For this review, take the finished solid that the model builds, in its own axes (mm). Coordinates: 2 decimals unless noted, no trailing zeros. Loops run counter-clockwise (first coordinate to the right, second up) from the corner with the lowest first, then second, coordinate; pieces in that order, holes last. Notation, with made-up numbers: (67.5, -31) - (81.5, -31) arc R24 ccw to (81.5, -14) - close; hole circle Ø3 at (35.25, -18.5). An arc over 180 degrees is marked (long way). Answer as a JSON object with one key per item and string values. Group by question number.
Item 1: To check wall thickness, follow line 1 (X direction, y = 1.15, z = -39); line 2 (Z direction, x = -18.5, y = 1.3); line 3 (X direction, y = 2.6, z = 25). State the ranges of each line that lie inside material, in increasing order.
Item 2: Clearance check with a flat-ended pin moving along its axis: pin 1 (1.5 mm diameter, centred on x = 70.5, y = 1, fed in from -Z). State where the tip first meets the part, or that it passes through.
Item 3: We need section B-B (y = 1.1). State how many separate pieces and enclosed holes the cut face has, then the cut area to 3 significant figures.
Item 4: We need section A-A (z = 12). Give the boundary of the cut face in (x, y).
from build123d import *

# Parameters (mm, degrees)
SKETCH1_R                = 100
SKETCH1_R_2              = 5
BOSS_EXTRUDE1_DEPTH      = 3
SKETCH2_W                = 5.2
SKETCH2_H                = 2.7
CUT_EXTRUDE1_DEPTH       = 4
CUT_EXTRUDE2_DEPTH       = 4
SKETCH4_W                = 5
SKETCH4_H                = 60
CUT_EXTRUDE3_DEPTH       = 4
FILLET3_R                = 10
FILLET2_R                = 1
SKETCH5_R                = 1.075
CUT_EXTRUDE4_DEPTH       = 4
SKETCH6_R                = 9
SKETCH6_R_2              = 1.1
CUT_EXTRUDE5_DEPTH       = 4
IR_HOLDER_HOLES_REACH    = 5
IR_HOLDER_HOLES_SKETCH_R = 1.5
PLATFORM_HOLES_REACH     = 5
PLATFORM_HOLES_SKETCH_R  = 1.5


with BuildPart() as part:
    # Sketch1 → Boss-Extrude1 (new body)
    with BuildSketch(Plane(origin=(0, 0, 0), x_dir=(1, 0, 0), z_dir=(0, 1, 0))):
        Circle(SKETCH1_R)
        Circle(SKETCH1_R_2, mode=Mode.SUBTRACT)
    extrude(amount=BOSS_EXTRUDE1_DEPTH)

    # Sketch2 → Cut-Extrude1 (cut, through all)
    with BuildSketch(Plane(origin=(0, 3, 0), x_dir=(1, 0, 0), z_dir=(0, 1, 0))):
        with Locations((-54.5, 37.95)):
            Rectangle(SKETCH2_W, SKETCH2_H)
        with Locations((-54.5, 28.45)):
            Rectangle(SKETCH2_W, SKETCH2_H)
        with Locations((-54.5, 4.75)):
            Rectangle(SKETCH2_W, SKETCH2_H)
        with Locations((-54.5, -4.75)):
            Rectangle(SKETCH2_W, SKETCH2_H)
        with Locations((-77.5, -4.75)):
            Rectangle(SKETCH2_W, SKETCH2_H)
        with Locations((-77.5, 4.75)):
            Rectangle(SKETCH2_W, SKETCH2_H)
        with Locations((54.5, 28.45)):
            Rectangle(SKETCH2_W, SKETCH2_H)
        with Locations((54.5, 37.95)):
            Rectangle(SKETCH2_W, SKETCH2_H)
        with Locations((77.5, 4.75)):
            Rectangle(SKETCH2_W, SKETCH2_H)
        with Locations((77.5, -4.75)):
            Rectangle(SKETCH2_W, SKETCH2_H)
        with Locations((54.5, -4.75)):
            Rectangle(SKETCH2_W, SKETCH2_H)
        with Locations((54.5, 4.75)):
            Rectangle(SKETCH2_W, SKETCH2_H)
    extrude(amount=-CUT_EXTRUDE1_DEPTH, mode=Mode.SUBTRACT)

    # Sketch3 → Cut-Extrude2 (cut, through all)
    with BuildSketch(Plane(origin=(0, 3, 0), x_dir=(1, 0, 0), z_dir=(0, 1, 0))):
        with BuildLine():
            ThreePointArc((67.534713296, 73.75), (0, 100), (-67.534713296, 73.75))
            Line((-67.534713296, 73.75), (67.534713296, 73.75))
        make_face()
        with BuildLine():
            Line((-85.1, -52.516568814), (-85.1, 52.516568814))
            ThreePointArc((-85.1, 52.516568814), (-100, 0), (-85.1, -52.516568814))
        make_face()
        with BuildLine():
            Line((67.534713296, -73.75), (-67.534713296, -73.75))
            ThreePointArc((-67.534713296, -73.75), (0, -100), (67.534713296, -73.75))
        make_face()
        with BuildLine():
            ThreePointArc((100, 0), (96.202910559, 27.294688128), (85.1, 52.516568814))
            Line((85.1, 52.516568814), (85.1, -52.516568814))
            ThreePointArc((85.1, -52.516568814), (96.202910559, -27.294688128), (100, 0))
        make_face()
    extrude(amount=-CUT_EXTRUDE2_DEPTH, mode=Mode.SUBTRACT)

    # Sketch4 → Cut-Extrude3 (cut, through all)
    with BuildSketch(Plane(origin=(0, 3, 0), x_dir=(1, 0, 0), z_dir=(0, 1, 0))):
        with Locations((-70.7, 0)):
            Rectangle(SKETCH4_W, SKETCH4_H)
        with Locations((70.7, 0)):
            Rectangle(SKETCH4_W, SKETCH4_H)
    extrude(amount=-CUT_EXTRUDE3_DEPTH, mode=Mode.SUBTRACT)

    # Fillet3
    fillet3_edges = [part.edges().sort_by_distance(p)[0] for p in [
        (-67.534713296, 1.5, -73.75),
        (67.534713296, 1.5, -73.75),
        (-85.1, 1.5, -52.516568814),
        (-85.1, 1.5, 52.516568814),
        (-67.534713296, 1.5, 73.75),
        (67.534713296, 1.5, 73.75),
        (85.1, 1.5, -52.516568814),
        (85.1, 1.5, 52.516568814),
    ]]
    fillet(fillet3_edges, radius=FILLET3_R)

    # Fillet2
    fillet2_edges = [part.edges().sort_by_distance(p)[0] for p in [
        (-73.2, 1.5, 30),
        (-73.2, 1.5, -30),
        (-68.2, 1.5, -30),
        (-68.2, 1.5, 30),
        (73.2, 1.5, -30),
        (73.2, 1.5, 30),
        (68.2, 1.5, 30),
        (68.2, 1.5, -30),
    ]]
    fillet(fillet2_edges, radius=FILLET2_R)

    # Sketch5 → Cut-Extrude4 (cut, through all)
    with BuildSketch(Plane(origin=(0, 3, 0), x_dir=(1, 0, 0), z_dir=(0, 1, 0))):
        with Locations((-54.5, 33.2)):
            Circle(SKETCH5_R)
        with Locations((-54.5, 0)):
            Circle(SKETCH5_R)
        with Locations((-77.5, 0)):
            Circle(SKETCH5_R)
        with Locations((77.5, 0)):
            Circle(SKETCH5_R)
        with Locations((54.5, 0)):
            Circle(SKETCH5_R)
        with Locations((54.5, 33.2)):
            Circle(SKETCH5_R)
    extrude(amount=-CUT_EXTRUDE4_DEPTH, mode=Mode.SUBTRACT)

    # Sketch6 → Cut-Extrude5 (cut, through all)
    with BuildSketch(Plane(origin=(0, 3, 0), x_dir=(1, 0, 0), z_dir=(0, 1, 0))):
        with Locations((0, 57.75)):
            Circle(SKETCH6_R)
        with Locations((0, 69.75)):
            Circle(SKETCH6_R_2)
        with Locations((12, 57.75)):
            Circle(SKETCH6_R_2)
        with Locations((0, 45.75)):
            Circle(SKETCH6_R_2)
        with Locations((-12, 57.75)):
            Circle(SKETCH6_R_2)
        with Locations((-12, -57.75)):
            Circle(SKETCH6_R_2)
        with Locations((0, -45.75)):
            Circle(SKETCH6_R_2)
        with Locations((12, -57.75)):
            Circle(SKETCH6_R_2)
        with Locations((0, -69.75)):
            Circle(SKETCH6_R_2)
        with Locations((0, -57.75)):
            Circle(SKETCH6_R)
    extrude(amount=-CUT_EXTRUDE5_DEPTH, mode=Mode.SUBTRACT)

    # IR Holder Holes Sketch → IR Holder Holes (cut, up to next)
    with BuildSketch(Plane(origin=(0, 3, 0), x_dir=(1, 0, 0), z_dir=(0, 1, 0)), mode=Mode.PRIVATE) as ir_holder_holes_sk1:
        with Locations((18.5, -65.75)):
            Circle(IR_HOLDER_HOLES_SKETCH_R)
    ir_holder_holes_tool1 = extrude(ir_holder_holes_sk1.sketch, amount=-IR_HOLDER_HOLES_REACH, mode=Mode.PRIVATE) & part.part
    add(ir_holder_holes_tool1.solids().sort_by_distance((18.5, 3, 65.75))[0], mode=Mode.SUBTRACT)
    # IR Holder Holes Sketch → IR Holder Holes (cut, up to next)
    with BuildSketch(Plane(origin=(0, 3, 0), x_dir=(1, 0, 0), z_dir=(0, 1, 0)), mode=Mode.PRIVATE) as ir_holder_holes_sk2:
        with Locations((18.5, -49.75)):
            Circle(IR_HOLDER_HOLES_SKETCH_R)
    ir_holder_holes_tool2 = extrude(ir_holder_holes_sk2.sketch, amount=-IR_HOLDER_HOLES_REACH, mode=Mode.PRIVATE) & part.part
    add(ir_holder_holes_tool2.solids().sort_by_distance((18.5, 3, 49.75))[0], mode=Mode.SUBTRACT)
    # IR Holder Holes Sketch → IR Holder Holes (cut, up to next)
    with BuildSketch(Plane(origin=(0, 3, 0), x_dir=(1, 0, 0), z_dir=(0, 1, 0)), mode=Mode.PRIVATE) as ir_holder_holes_sk3:
        with Locations((-18.5, -65.75)):
            Circle(IR_HOLDER_HOLES_SKETCH_R)
    ir_holder_holes_tool3 = extrude(ir_holder_holes_sk3.sketch, amount=-IR_HOLDER_HOLES_REACH, mode=Mode.PRIVATE) & part.part
    add(ir_holder_holes_tool3.solids().sort_by_distance((-18.5, 3, 65.75))[0], mode=Mode.SUBTRACT)
    # IR Holder Holes Sketch → IR Holder Holes (cut, up to next)
    with BuildSketch(Plane(origin=(0, 3, 0), x_dir=(1, 0, 0), z_dir=(0, 1, 0)), mode=Mode.PRIVATE) as ir_holder_holes_sk4:
        with Locations((-18.5, -49.75)):
            Circle(IR_HOLDER_HOLES_SKETCH_R)
    ir_holder_holes_tool4 = extrude(ir_holder_holes_sk4.sketch, amount=-IR_HOLDER_HOLES_REACH, mode=Mode.PRIVATE) & part.part
    add(ir_holder_holes_tool4.solids().sort_by_distance((-18.5, 3, 49.75))[0], mode=Mode.SUBTRACT)

    # Platform Holes Sketch → Platform Holes (cut, up to next)
    with BuildSketch(Plane(origin=(0, 3, 0), x_dir=(1, 0, 0), z_dir=(0, 1, 0)), mode=Mode.PRIVATE) as platform_holes_sk1:
        with Locations((-66.529028798, 66.25)):
            Circle(PLATFORM_HOLES_SKETCH_R)
    platform_holes_tool1 = extrude(platform_holes_sk1.sketch, amount=-PLATFORM_HOLES_REACH, mode=Mode.PRIVATE) & part.part
    add(platform_holes_tool1.solids().sort_by_distance((-66.529029, 3, -66.25))[0], mode=Mode.SUBTRACT)
    # Platform Holes Sketch → Platform Holes (cut, up to next)
    with BuildSketch(Plane(origin=(0, 3, 0), x_dir=(1, 0, 0), z_dir=(0, 1, 0)), mode=Mode.PRIVATE) as platform_holes_sk2:
        with Locations((66.470971202, 66.25)):
            Circle(PLATFORM_HOLES_SKETCH_R)
    platform_holes_tool2 = extrude(platform_holes_sk2.sketch, amount=-PLATFORM_HOLES_REACH, mode=Mode.PRIVATE) & part.part
    add(platform_holes_tool2.solids().sort_by_distance((66.470971, 3, -66.25))[0], mode=Mode.SUBTRACT)
    # Platform Holes Sketch → Platform Holes (cut, up to next)
    with BuildSketch(Plane(origin=(0, 3, 0), x_dir=(1, 0, 0), z_dir=(0, 1, 0)), mode=Mode.PRIVATE) as platform_holes_sk3:
        with Locations((-66.529028798, -66.25)):
            Circle(PLATFORM_HOLES_SKETCH_R)
    platform_holes_tool3 = extrude(platform_holes_sk3.sketch, amount=-PLATFORM_HOLES_REACH, mode=Mode.PRIVATE) & part.part
    add(platform_holes_tool3.solids().sort_by_distance((-66.529029, 3, 66.25))[0], mode=Mode.SUBTRACT)
    # Platform Holes Sketch → Platform Holes (cut, up to next)
    with BuildSketch(Plane(origin=(0, 3, 0), x_dir=(1, 0, 0), z_dir=(0, 1, 0)), mode=Mode.PRIVATE) as platform_holes_sk4:
        with Locations((66.529028798, -66.25)):
            Circle(PLATFORM_HOLES_SKETCH_R)
    platform_holes_tool4 = extrude(platform_holes_sk4.sketch, amount=-PLATFORM_HOLES_REACH, mode=Mode.PRIVATE) & part.part
    add(platform_holes_tool4.solids().sort_by_distance((66.529029, 3, 66.25))[0], mode=Mode.SUBTRACT)


solid = part.part
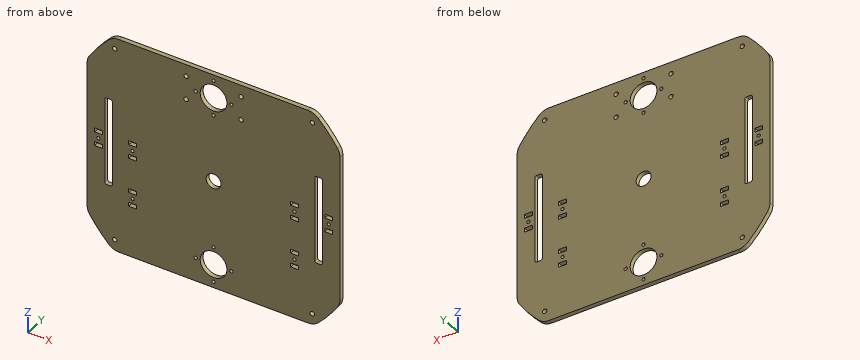
Check sheet entries:
{
 "1": {"line 1": "x = -85.1 to -57.1, -51.9 to 51.9, 57.1 to 85.1", "line 2": "z = -73.75 to 48.25, 51.25 to 64.25, 67.25 to 73.75", "line 3": "x = -85.1 to -73.2, -68.2 to 68.2, 73.2 to 85.1"},
 "2": {"pin 1": "stops at z = -71.58"},
 "3": {"separate pieces": "1", "enclosed holes": "39", "area": "23,000 mm2"},
 "4": {"outline": "(-85.1, 0) - (-73.2, 0) - (-73.2, 3) - (-85.1, 3) - close; (-68.2, 0) - (68.2, 0) - (68.2, 3) - (-68.2, 3) - close; (73.2, 0) - (85.1, 0) - (85.1, 3) - (73.2, 3) - close"}
}
